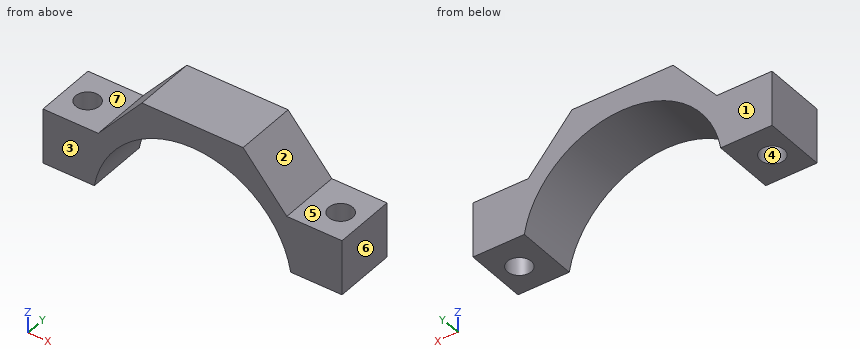
from build123d import *

# Parameters (mm, degrees)
F0_R     = 27.5
F1_DEPTH = 38.1
F2_W     = 19.05
F2_H     = 5.08
F3_DEPTH = 38.1
F5_D     = 6.6
F6_W     = 88.9
F6_H     = 38.1
F7_DEPTH = 36.83
F8_W     = 82.55
F8_H     = 29.21
F9_DEPTH = 20.955


with BuildPart() as f1:
    # F0 (on Front) → F1 (new body)
    with BuildSketch(Plane.XZ):
        Polygon((-44.45, 0), (0, 0), (44.45, 0), (44.45, 17.78), (41.275, 19.05), (41.275, 52.07), (26.035, 52.07), (13.97, 66.04), (0, 66.04), (-13.97, 66.04), (-26.035, 52.07), (-41.275, 52.07), (-41.275, 19.05), (-44.45, 17.78), align=None)
        with Locations((0, 32.19)):
            Circle(F0_R, mode=Mode.SUBTRACT)
    extrude(amount=F1_DEPTH)

    # F2 (on face) → F3 (cut, through all)
    with BuildSketch(Plane.XZ.offset(38.1)):
        with Locations((-31.75, 34.29)):
            Rectangle(F2_W, F2_H)
    extrude(amount=-F3_DEPTH, mode=Mode.SUBTRACT)

    # F5 (through all)
    with Locations(Plane.XY.offset(52.07)):
        with Locations((-34.925, -8.89), (-34.925, -29.21), (34.925, -8.89), (34.925, -29.21)):
            Hole(F5_D / 2)

    # F6 (on face) → F7 (cut, through all)
    with BuildSketch(Plane(origin=(0, 0, 0), x_dir=(1, 0, 0), z_dir=(0, 0, -1))):
        with Locations((0, 19.05)):
            Rectangle(F6_W, F6_H)
    extrude(amount=-F7_DEPTH, mode=Mode.SUBTRACT)

    # F8 (on face) → F9 (cut)
    with BuildSketch(Plane.XZ.offset(38.1)):
        with Locations((0, 51.435)):
            Rectangle(F8_W, F8_H)
    extrude(amount=-F9_DEPTH, mode=Mode.SUBTRACT)


solid = f1.part
Read the model definition and answer for the solid it produces. Units are mm, in the model's axes. Face numbers are marked on the shaded views. A direction names the side the tool comes from. Give positions to 0.01 mm unless a question says otherwise; leave off trailing zeros. Write each loop counter-clockwise with the first axis right and the second up, starting at its lowest first coordinate (ties: lowest second). Pieces come first, ordered by that corner, then holes. Notation, with made-up numbers: (-30.75, -9) - (4.25, -9) arc R19 cw to (4.25, 13) - close; hole circle Ø3 at (-23.5, -19). An arc over 180 degrees is marked (long way). Use CSV: the item, a comma, the result in double quotes. Start each with the question number.
Item 1: For the marked faces 5, 6 and 7, determine the directions among +Z, -Z, +X, -X, +Y, -Y from which every point of the face is accessible in a straight line to the end or side of a thin tool.
Item 2: Flat-ended cylindrical pins translate along their axes: P1, Ø5, axis at x = 32.5, y = -5, coming from the +Z side; P2, Ø8, axis at y = -5.5, z = 59.5, coming from the +X side. Find the tip coordinate at first contact, or state that the pin passes through.
Item 3: The part is cut by section C-C, the plane y = -3.5. Give the vertices of the cut face in (x, z) (3 decimals), and give its area (3 significant figures).
Item 4: The part is cut by section B-B, the plane z = 56.5. Give the vertices of the cut face in (x, y) (3 decimals).
Item 5: The mould has two halves that part along Y. Classify the marked faces 1, 2, 3 and 4: pulls with the +Y half, pulls with the -Y half, needs draft (parallel to the pull), parting line crosses it, or undercut.
Item 6: The part is cut by section D-D, the plane x = 5.5. Give the vertices of the cut face in (y, z) (3 decimals).
Item 7: Consider line 1 (X direction, y = -7.75, z = 44.25) (1 decimal); line 2 (X direction, y = -7.5, z = 46.5) (3 decimals); line 3 (Y direction, x = 35, z = 41) (3 decimals). Determine where each line is inside the solid, lowest interval first.
Item 8: The part is cut by section A-A, the plane y = -8.89. Give the vertices of the cut face in (x, z) (3 decimals).
Taken from the geometry:
1,face 5,"+Z, +X, +Y, -Y"
1,face 6,"+Z, -Z, +X, +Y, -Y"
1,face 7,"+Z, -X, +Y, -Y"
2,P1,"z = 52.07"
2,P2,"x = 23.07"
3,outline,"(-41.275, 36.83) - (-27.106, 36.83) arc R27.5 cw to (27.106, 36.83) - (41.275, 36.83) - (41.275, 52.07) - (26.035, 52.07) - (13.97, 66.04) - (-13.97, 66.04) - (-26.035, 52.07) - (-41.275, 52.07) - close"
3,area,"883 mm2"
4,outline,"(-22.209, -17.145) - (-12.856, -17.145) - (-12.856, 0) - (-22.209, 0) - close; (12.856, -17.145) - (22.209, -17.145) - (22.209, 0) - (12.856, 0) - close"
5,face 1,"pulls with the +Y half"
5,face 2,"needs draft"
5,face 3,"pulls with the -Y half"
5,face 4,"undercut"
6,outline,"(-17.145, 59.134) - (0, 59.134) - (0, 66.04) - (-17.145, 66.04) - close"
7,line 1,"-41.3 to -38, -31.8 to -24.7, 24.7 to 31.8, 38 to 41.3"
7,line 2,"-41.275 to -37.918, -31.932 to -23.483, 23.483 to 31.932, 37.918 to 41.275"
7,line 3,"-17.145 to -12.189, -5.591 to 0"
8,outline,"(-41.275, 36.83) - (-38.225, 36.83) - (-38.225, 52.07) - (-41.275, 52.07) - close; (-31.625, 36.83) - (-27.106, 36.83) arc R27.5 cw to (27.106, 36.83) - (31.625, 36.83) - (31.625, 52.07) - (26.035, 52.07) - (13.97, 66.04) - (-13.97, 66.04) - (-26.035, 52.07) - (-31.625, 52.07) - close; (38.225, 36.83) - (41.275, 36.83) - (41.275, 52.07) - (38.225, 52.07) - close"
